```python
from build123d import *
from build123d.topology import SkipClean

# Parameters (mm, degrees)
SKETCH1_W           = 7
SKETCH1_H           = 7
BOSS_EXTRUDE1_DEPTH = 3.2
CHAMFER1_SIZE       = 1.5
FILLET1_R           = 3.5
CHAMFER2_SIZE       = 3.4
SKETCH3_R           = 2
BOSS_EXTRUDE2_DEPTH = 4.25
BOSS_EXTRUDE3_DEPTH = 1.85
BOSS_EXTRUDE4_DEPTH = 1.85


with BuildPart() as part:
    # Sketch1 → Boss-Extrude1 (new body)
    with BuildSketch(Plane(origin=(0, 0, 0), x_dir=(0, 0, -1), z_dir=(1, 0, 0))):
        Polygon((6.9, 3.5), (6.9, 6.9), (-6.9, 6.9), (-6.9, -6.9), (6.9, -6.9), (6.9, -3.5), (19.9, -3.5), (19.9, 3.5), align=None)
        Rectangle(SKETCH1_W, SKETCH1_H, mode=Mode.SUBTRACT)
    extrude(amount=BOSS_EXTRUDE1_DEPTH)

    # Chamfer1
    chamfer1_edges = [part.edges().sort_by_distance(p)[0] for p in [
        (1.6, -3.5, -3.5),
        (1.6, 3.5, -3.5),
        (1.6, 3.5, 3.5),
        (1.6, -3.5, 3.5),
    ]]
    chamfer(chamfer1_edges, length=CHAMFER1_SIZE)

    # Fillet1
    fillet1_edges = [part.edges().sort_by_distance(p)[0] for p in [
        (1.6, -3.5, -19.9),
        (1.6, 3.5, -19.9),
    ]]
    fillet(fillet1_edges, radius=FILLET1_R - 0.0001)  # a hair under: the kernel refuses the full size

    # Chamfer2
    chamfer2_edges = [part.edges().sort_by_distance(p)[0] for p in [
        (1.6, -6.9, -6.9),
        (1.6, -6.9, 6.9),
        (1.6, 6.9, 6.9),
        (1.6, 6.9, -6.9),
    ]]
    chamfer(chamfer2_edges, length=CHAMFER2_SIZE - 0.0001)  # a hair under: the kernel refuses the full size

    # Sketch3 → Boss-Extrude2 (add)
    with BuildSketch(Plane.ZY):
        with Locations(Location((-16.4, 0, 0), (0, 0, 180))):
            Circle(SKETCH3_R)
    extrude(amount=BOSS_EXTRUDE2_DEPTH)

    # Sketch4 → Boss-Extrude3 (add)
    with BuildSketch(Plane(origin=(3.2, 0, 0), x_dir=(0, 0, -1), z_dir=(1, 0, 0))):
        with BuildLine():
            Line((6.9, 2.234550653), (15.178957615, 1.979760355))
            ThreePointArc((15.178957615, 1.979760355), (16.745857217, 0), (15.178957615, -1.979760355))
            Line((15.178957615, -1.979760355), (6.9, -2.234550653))
            Line((6.9, -2.234550653), (5.852935753, -3.314334724))
            Line((5.852935753, -3.314334724), (15.305699084, -3.023419792))
            ThreePointArc((15.305699084, -3.023419792), (17.792921464, 0), (15.305699084, 3.023419792))
            Line((15.305699084, 3.023419792), (5.852935753, 3.314334724))
            Line((5.852935753, 3.314334724), (6.9, 2.234550653))
        make_face()
    extrude(amount=BOSS_EXTRUDE3_DEPTH)

    # Sketch5 → Boss-Extrude4 (add)
    with SkipClean():  # the faces are left unmerged after this step: merging them gives an invalid solid
        with BuildSketch(Plane(origin=(3.2, 0, 0), x_dir=(0, 0, -1), z_dir=(1, 0, 0))):
            with BuildLine():
                Line((-6.9, -3.5), (-3.5, -6.9))
                Line((-3.5, -6.9), (3.5, -6.9))
                Line((3.5, -6.9), (6.9, -3.5))
                Line((6.9, -3.5), (16.4, -3.5))
                ThreePointArc((16.4, -3.5), (18.874873734, -2.474873734), (19.9, 0))
                ThreePointArc((19.9, 0), (18.874873734, 2.474873734), (16.4, 3.5))
                Line((16.4, 3.5), (6.9, 3.5))
                Line((6.9, 3.5), (3.5, 6.9))
                Line((3.5, 6.9), (-3.5, 6.9))
                Line((-3.5, 6.9), (-6.9, 3.5))
                Line((-6.9, 3.5), (-6.9, -3.5))
            make_face()
            with BuildLine():
                Line((5.852935753, -3.314334724), (2, -3.5))
                Line((2, -3.5), (-2, -3.5))
                Line((-2, -3.5), (-3.5, -2))
                Line((-3.5, -2), (-3.5, 2))
                Line((-3.5, 2), (-2, 3.5))
                Line((-2, 3.5), (2, 3.5))
                Line((2, 3.5), (5.852935753, 3.314334724))
                Line((5.852935753, 3.314334724), (15.305699084, 3.023419792))
                ThreePointArc((15.305699084, 3.023419792), (17.792921464, 0), (15.305699084, -3.023419792))
                Line((15.305699084, -3.023419792), (5.852935753, -3.314334724))
            make_face(mode=Mode.SUBTRACT)
        extrude(amount=BOSS_EXTRUDE4_DEPTH)


solid = part.part
```
Here's how the part is built. I have some questions about the finished solid (model axes, mm). A direction names the side the tool comes from. Round coordinates to 2 decimals unless told otherwise and drop trailing zeros. Order: outer loops, then holes, each group sorted by start corner. A loop starts at its lowest first (then second) coordinate and runs counter-clockwise, first axis right, second up. Notation, with made-up numbers: M -3.75,78.25 L 7.25,78.25 A15 ccw 7.25,103.25 Z; hole C 35.25,26 d2. An arc over 180 degrees is marked long. Use CSV: the item, a comma, the result in double quotes.
1) On a 3-axis mill with a long thin cutter (end or side, diameter ignored), from which of +Z, -Z, +X, -X, +Y, -Y can I reach the whole of each face in a straight line? I mean faces 1 (the flat face through (3.2, 0, -9)), 2 (the cylindrical face through (1.62, -2.45, -18.9)), 3 (the flat face through (2, 0, -3.5)). Say none if no direction works.
Taken from the geometry:
face 1,"+X"
face 2,"-Z, +X, -X, -Y"
face 3,"+X, -X"
2) I want a section at A-A (x = 4.5). List the corners of the cut face in (y, z) for me.
Taken from the geometry:
outline,"M -6.9,-3.5 L -3.5,-6.9 L -3.5,-16.4 A3.5 ccw 3.5,-16.4 L 3.5,-6.9 L 6.9,-3.5 L 6.9,3.5 L 3.5,6.9 L -3.5,6.9 L -6.9,3.5 Z; hole M -3.5,-2 L -3.31,-5.85 L -2.23,-6.9 L -1.98,-15.18 A2.03 ccw 1.98,-15.18 L 2.23,-6.9 L 3.31,-5.85 L 3.5,-2 L 3.5,2 L 2,3.5 L -2,3.5 L -3.5,2 Z"
3) If we mould it in two halves opening along Y, with no side actions, what happens to faces 4 (the flat face through (2.5, -2.8, 2.7)), 5 (the flat face through (2, -3.5, -12)), 6 (the cylindrical face through (-2.095, -0.601, -18.308))? For each: pulls with the +Y half, pulls with the -Y half, needs draft (parallel to the pull), parting line crosses it, or undercut.
Taken from the geometry:
face 4,"undercut"
face 5,"pulls with the -Y half"
face 6,"parting line crosses it"
4) I want a section at B-B (z = 1). List the corners of the cut face in (x, y) for me, then the cut area to 3 significant figures.
Taken from the geometry:
outline,"M 0,-6.9 L 5.05,-6.9 L 5.05,-3.5 L 0,-3.5 Z; M 0,3.5 L 5.05,3.5 L 5.05,6.9 L 0,6.9 Z"
area,"34.3 mm^2"
5) I need wall thicknesses on line 1 along Y through (x, z) = (2.5, 1.75); line 2 along X through (y, z) = (-4.75, -0.25); line 3 along X through (y, z) = (-1.75, -11). Which ranges of each line are inside material? Lowest first, please. Write a range as [from, to].
Taken from the geometry:
line 1,"[-6.9, -3.5], [3.5, 6.9]"
line 2,"[0, 5.05]"
line 3,"[0, 3.2]"
6) I'm going to push flat-ended pins straight in: P1, Ø2.5, axis at x = 3.5, z = -9.5, coming from the +Y side; P2, Ø1, axis at y = 0, z = -4, coming from the +X side; P3, Ø2.5, axis at x = 2.5, z = -11.5, coming from the -Y side. Where does each tip first touch, or does it pass through?
Taken from the geometry:
P1,"y = 3.5"
P2,"x = 3.2"
P3,"y = -3.5"
